Read the model definition and answer for the solid it produces. Units are mm, in the model's axes. A direction names the side the tool comes from. Give positions to 0.01 mm unless a question says otherwise; leave off trailing zeros. Order: outer loops, then holes, each group sorted by start corner. A loop starts at its lowest first (then second) coordinate and runs counter-clockwise, first axis right, second up. Notation, with made-up numbers: M -1,-9 L 55,-9 A19 ccw 55,16 Z; hole C -8.75,83 d10. An arc over 180 degrees is marked long. One line per item, written item: value.
from build123d import *

# Parameters (mm, degrees)
SKETCH1_R           = 1.25
BOSS_EXTRUDE1_DEPTH = 7
SKETCH2_W           = 16.7
SKETCH2_H           = 20.32
CUT_EXTRUDE1_DEPTH  = 5
SKETCH3_R           = 1.25
CUT_EXTRUDE2_DEPTH  = 2
CHAMFER1_SIZE       = 1
FILLET1_R           = 0.5
FILLET2_R           = 0.5


with BuildPart() as part:
    # Sketch1 → Boss-Extrude1 (new body)
    with BuildSketch(Plane(origin=(0, -16.169464744, 0), x_dir=(1, 0, 0), z_dir=(0, 1, 0))):
        with BuildLine():
            Line((-127.05696299, -71.463712198), (-127.05696299, -86.703712198))
            ThreePointArc((-127.05696299, -86.703712198), (-127.800911766, -88.499763423), (-129.59696299, -89.243712198))
            Line((-129.59696299, -89.243712198), (-151.18696299, -89.243712198))
            ThreePointArc((-151.18696299, -89.243712198), (-152.983014214, -88.499763423), (-153.72696299, -86.703712198))
            Line((-153.72696299, -86.703712198), (-153.72696299, -71.463712198))
            ThreePointArc((-153.72696299, -71.463712198), (-152.983014214, -69.667660974), (-151.18696299, -68.923712198))
            Line((-151.18696299, -68.923712198), (-129.59696299, -68.923712198))
            ThreePointArc((-129.59696299, -68.923712198), (-127.800911766, -69.667660974), (-127.05696299, -71.463712198))
        make_face()
        with Locations((-151.18696299, -71.463712198)):
            Circle(SKETCH1_R, mode=Mode.SUBTRACT)
        with Locations((-151.18696299, -86.703712198)):
            Circle(SKETCH1_R, mode=Mode.SUBTRACT)
        with Locations((-129.59696299, -86.703712198)):
            Circle(SKETCH1_R, mode=Mode.SUBTRACT)
        with Locations((-129.59696299, -71.463712198)):
            Circle(SKETCH1_R, mode=Mode.SUBTRACT)
    extrude(amount=BOSS_EXTRUDE1_DEPTH)

    # Sketch2 → Cut-Extrude1 (cut)
    with BuildSketch(Plane.XZ.offset(16.169464744)):
        with Locations((-140.39196299, 79.083712198)):
            Rectangle(SKETCH2_W, SKETCH2_H)
    extrude(amount=-CUT_EXTRUDE1_DEPTH, mode=Mode.SUBTRACT)

    # Sketch3 → Cut-Extrude2 (cut)
    with BuildSketch(Plane(origin=(0, -9.169464744, 0), x_dir=(1, 0, 0), z_dir=(0, 1, 0))):
        with BuildLine():
            Line((-131.84696299, -86.703712198), (-131.84696299, -89.243712198))
            Line((-131.84696299, -89.243712198), (-129.59696299, -89.243712198))
            ThreePointArc((-129.59696299, -89.243712198), (-127.800911766, -88.499763423), (-127.05696299, -86.703712198))
            Line((-127.05696299, -86.703712198), (-127.05696299, -84.453712198))
            Line((-127.05696299, -84.453712198), (-129.59696299, -84.453712198))
            ThreePointArc((-129.59696299, -84.453712198), (-131.187953248, -85.112721941), (-131.84696299, -86.703712198))
        make_face()
        with Locations((-129.59696299, -86.703712198)):
            Circle(SKETCH3_R, mode=Mode.SUBTRACT)
        with BuildLine():
            Line((-151.18696299, -89.243712198), (-148.93696299, -89.243712198))
            Line((-148.93696299, -89.243712198), (-148.93696299, -86.703712198))
            ThreePointArc((-148.93696299, -86.703712198), (-149.595972732, -85.112721941), (-151.18696299, -84.453712198))
            Line((-151.18696299, -84.453712198), (-153.72696299, -84.453712198))
            Line((-153.72696299, -84.453712198), (-153.72696299, -86.703712198))
            ThreePointArc((-153.72696299, -86.703712198), (-152.983014214, -88.499763423), (-151.18696299, -89.243712198))
        make_face()
        with Locations((-151.18696299, -86.703712198)):
            Circle(SKETCH3_R, mode=Mode.SUBTRACT)
        with BuildLine():
            Line((-153.72696299, -71.463712198), (-153.72696299, -73.713712198))
            Line((-153.72696299, -73.713712198), (-151.18696299, -73.713712198))
            ThreePointArc((-151.18696299, -73.713712198), (-149.595972732, -73.054702456), (-148.93696299, -71.463712198))
            Line((-148.93696299, -71.463712198), (-148.93696299, -68.923712198))
            Line((-148.93696299, -68.923712198), (-151.18696299, -68.923712198))
            ThreePointArc((-151.18696299, -68.923712198), (-152.983014214, -69.667660974), (-153.72696299, -71.463712198))
        make_face()
        with Locations((-151.18696299, -71.463712198)):
            Circle(SKETCH3_R, mode=Mode.SUBTRACT)
        with BuildLine():
            Line((-129.59696299, -73.713712198), (-127.05696299, -73.713712198))
            Line((-127.05696299, -73.713712198), (-127.05696299, -71.463712198))
            ThreePointArc((-127.05696299, -71.463712198), (-127.800911766, -69.667660974), (-129.59696299, -68.923712198))
            Line((-129.59696299, -68.923712198), (-131.84696299, -68.923712198))
            Line((-131.84696299, -68.923712198), (-131.84696299, -71.463712198))
            ThreePointArc((-131.84696299, -71.463712198), (-131.187953248, -73.054702456), (-129.59696299, -73.713712198))
        make_face()
        with Locations((-129.59696299, -71.463712198)):
            Circle(SKETCH3_R, mode=Mode.SUBTRACT)
    extrude(amount=-CUT_EXTRUDE2_DEPTH, mode=Mode.SUBTRACT)

    # Chamfer1
    chamfer1_edges = [part.edges().sort_by_distance(p)[0] for p in [
        (-127.05696299, -9.169464744, 79.083712198),
        (-153.72696299, -9.169464744, 79.083712198),
        (-140.39196299, -9.169464744, 68.923712198),
        (-140.39196299, -9.169464744, 89.243712198),
    ]]
    chamfer(chamfer1_edges, length=CHAMFER1_SIZE)

    # Fillet1
    fillet1_edges = [part.edges().sort_by_distance(p)[0] for p in [
        (-148.74196299, -11.169464744, 79.083712198),
        (-132.04196299, -11.169464744, 79.083712198),
    ]]
    fillet(fillet1_edges, radius=FILLET1_R)

    # Fillet2
    fillet2_edges = [part.edges().sort_by_distance(p)[0] for p in [
        (-148.93696299, -11.169464744, 87.973712198),
        (-152.45696299, -11.169464744, 84.453712198),
        (-149.595972732, -11.169464744, 85.112721941),
        (-131.187953248, -11.169464744, 85.112721941),
        (-128.32696299, -11.169464744, 84.453712198),
        (-131.84696299, -11.169464744, 87.973712198),
        (-131.84696299, -11.169464744, 70.193712198),
        (-128.32696299, -11.169464744, 73.713712198),
        (-131.187953248, -11.169464744, 73.054702456),
        (-149.595972732, -11.169464744, 73.054702456),
        (-152.45696299, -11.169464744, 73.713712198),
        (-148.93696299, -11.169464744, 70.193712198),
    ]]
    fillet(fillet2_edges, radius=FILLET2_R)


solid = part.part
1) Find section B-B, the plane z = 74. Write down the section's boundary in (x, y).
Reported:
outline: M -153.73,-16.17 L -148.74,-16.17 L -148.74,-11.67 A0.5 cw -148.24,-11.17 L -132.54,-11.17 A0.5 cw -132.04,-11.67 L -132.04,-16.17 L -127.06,-16.17 L -127.06,-10.17 L -128.06,-9.17 L -152.73,-9.17 L -153.73,-10.17 Z
2) Determine the mould class of faces 6 (the face through (-127.057, -13, 79)), 7 (the face through (-152.96, -13.7, 88.52)), 8 (the face through (-148.742, -14, 79)) for opening direction X: +X half, -X half, draft (parallel to the pull), parting line (faces both ways), or undercut.
Reported:
face 6: +X half
face 7: -X half
face 8: undercut
3) Which of the six approach directions +Z, -Z, +X, -X, +Y, -Y give full straight-line access (tool end or side, diameter ignored) to faces 1 (the face through (-152.18, -13.7, 72.22)), 2 (the face through (-153, -11.169, 87)), 3 (the face through (-131.17, -9.909, 85.095)), 4 (the face through (-148.937, -10, 70)), 5 (the face through (-153.003, -13.704, 69.688))?
Reported:
face 1: +Y, -Y
face 2: +Z, -X, +Y
face 3: +Z, +X, +Y
face 4: -Z, -X, +Y
face 5: -Z, -X, +Y, -Y
4) Find section C-C, the plane x = -128.75. Write down the section's boundary in (y, z), plus the area to 3 significant figures.
Reported:
outline: M -16.17,69.07 L -11.17,69.07 L -11.17,70.54 L -16.17,70.54 Z; M -16.17,72.38 L -11.17,72.38 L -11.17,73.21 A0.5 cw -10.67,73.71 L -9.17,73.71 L -9.17,84.45 L -10.67,84.45 A0.5 cw -11.17,84.95 L -11.17,85.78 L -16.17,85.78 Z; M -16.17,87.62 L -11.17,87.62 L -11.17,89.1 L -16.17,89.1 Z
area: 103 mm^2
5) Find section A-A, the plane y = -15.5. Write down the section's boundary in (x, z).
Reported:
outline: M -153.73,71.46 A2.54 ccw -151.19,68.92 L -148.74,68.92 L -148.74,89.24 L -151.19,89.24 A2.54 ccw -153.73,86.7 Z; M -132.04,68.92 L -129.6,68.92 A2.54 ccw -127.06,71.46 L -127.06,86.7 A2.54 ccw -129.6,89.24 L -132.04,89.24 Z; hole C -151.19,71.46 d2.5; hole C -151.19,86.7 d2.5; hole C -129.6,71.46 d2.5; hole C -129.6,86.7 d2.5
6) Consider probe 1 along Z at (x, y) = (-129.5, -14); probe 2 along X at (y, z) = (-14.5, 81); probe 3 along X at (y, z) = (-11.75, 87.5) (3 decimals). Determine where each line is inside the solid, lowest interval first.
Reported:
probe 1: z = 68.93 to 70.22, 72.71 to 85.46, 87.95 to 89.24
probe 2: x = -153.73 to -148.74, -132.04 to -127.06
probe 3: x = -153.599 to -152.151, -150.223 to -148.742, -132.042 to -130.561, -128.633 to -127.185
7) Find section D-D, the plane z = 87.5. Write down the section's boundary in (x, y) (3 decimals), plus the area to 3 significant figures.
Reported:
outline: M -153.599,-16.169 L -152.151,-16.169 L -152.151,-11.169 L -153.599,-11.169 Z; M -150.223,-16.169 L -148.742,-16.169 L -148.742,-11.669 A0.5 cw -148.242,-11.169 L -132.542,-11.169 A0.5 cw -132.042,-11.669 L -132.042,-16.169 L -130.561,-16.169 L -130.561,-11.169 L -131.347,-11.169 A0.5 cw -131.847,-10.669 L -131.847,-9.169 L -148.937,-9.169 L -148.937,-10.669 A0.5 cw -149.437,-11.169 L -150.223,-11.169 Z; M -128.633,-16.169 L -127.185,-16.169 L -127.185,-11.169 L -128.633,-11.169 Z
area: 63.7 mm^2
8) Each of these flat-tipped pins is pushed along its axis until it touches: pin 1 Ø1.2 at (x, y) = (-153, -9.5) entering from +Z; pin 2 Ø0.5 at (y, z) = (-10, 70) entering from -X; pin 3 Ø1.7 at (y, z) = (-10, 70.5) entering from +X. Where does it stop, or does it pass through?
Reported:
pin 1: stops at z = 84.45
pin 2: stops at x = -148.94
pin 3: stops at x = -131.81
